Input: dimensioned drawing with shaded views. Units: mm. Origin: part minimum x, y, z. A direction names the side the tool comes from. Coordinates: 2 decimals unless noted, no trailing zeros. Order: outer loops, then holes, each group sorted by start corner. A loop starts at its lowest first (then second) coordinate and runs counter-clockwise, first axis right, second up. Notation, with made-up numbers: (55.5, 34) -> (90.5, 34) arc R17 ccw to (90.5, 43) -> close; hole circle Ø7 at (-16.5, -12). An arc over 180 degrees is marked (long way). Answer as CSV lines item,"result".
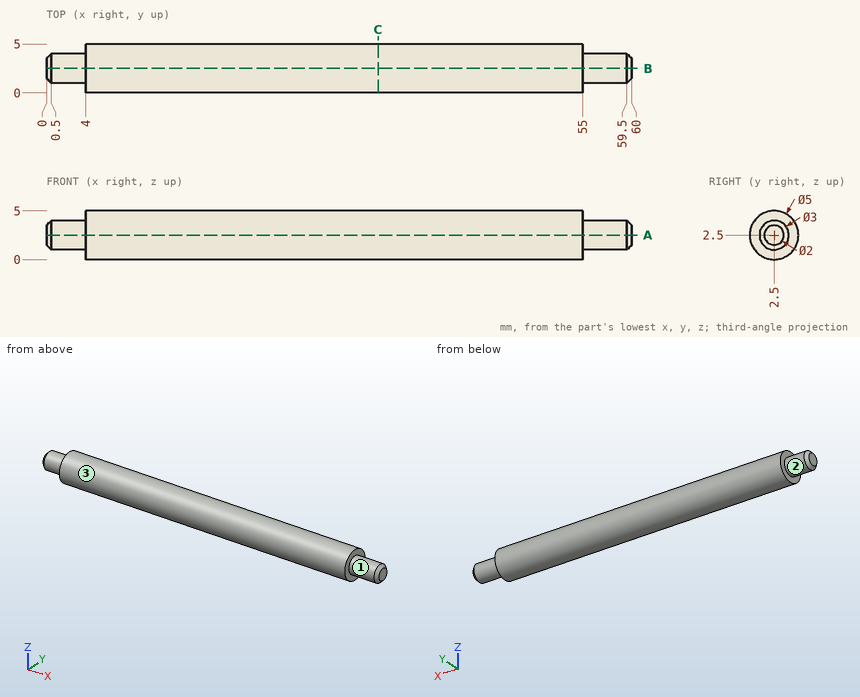
1. Contact query for a flat-ended pin moving along its axis: pin 1 (2 mm diameter, centred on x = 11.5, z = 4.5, fed in from -Y). Output: stop coordinate, or through.
Findings:
pin 1,"stops at y = 0.21"
2. Ray query, line 1 along X through (y, z) = (3.5, 3.65); line 2 along Z through (x, y) = (14.5, 4.5); line 3 along Y through (x, z) = (15, 2.75). Return the intervals inside material, ascending.
Findings:
line 1,"x = 4 to 55"
line 2,"z = 1 to 4"
line 3,"y = 0.01 to 4.99"
3. Cut plane C-C (x = 34). Return the cut outline in (y, z).
Findings:
outline,"circle Ø5 at (2.5, 2.5)"
4. Cut plane A-A (z = 2.5). Return the cut outline in (x, y).
Findings:
outline,"(0, 1.5) -> (0.5, 1) -> (4, 1) -> (4, 0) -> (55, 0) -> (55, 1) -> (59.5, 1) -> (60, 1.5) -> (60, 3.5) -> (59.5, 4) -> (55, 4) -> (55, 5) -> (4, 5) -> (4, 4) -> (0.5, 4) -> (0, 3.5) -> close"
5. Reachability of the marked faces 1, 2 and 3 from +Z, -Z, +X, -X, +Y, -Y: full face, straight path, thin tool, end or side. Return the list, or none.
Findings:
face 1,"+X"
face 2,"-X"
face 3,"+X, -X"
